The listing builds one solid part. Answer for the finished solid, in the listing's coordinates (mm). A direction names the side the tool comes from. Coordinates: 2 decimals unless noted, no trailing zeros. Write each loop counter-clockwise with the first axis right and the second up, starting at its lowest first coordinate (ties: lowest second). Pieces come first, ordered by that corner, then holes. Notation, with made-up numbers: M 54,22 L 95,22 A12 cw 95,45 Z; hole C 79,37.5 d11. An arc over 180 degrees is marked long. Write item = value, one per line. Start each with the question number.
```python
from build123d import *

# Parameters (mm, degrees)
SKETCH1_W                      = 65
SKETCH1_H                      = 32
EXTRUDE1_DEPTH                 = 6.35
CBORE_FOR_M4_SHCS1_D           = 4.5
CBORE_FOR_M4_SHCS1_CBORE_D     = 8
CBORE_FOR_M4_SHCS1_CBORE_DEPTH = 4
LPATTERN2_COUNT                = 2
LPATTERN2_PITCH                = 58
LPATTERN2_COUNT_DIR2           = 2
LPATTERN2_PITCH_DIR2           = 25
CBORE_FOR_M3_SHCS1_D           = 3.4
CBORE_FOR_M3_SHCS1_CBORE_D     = 6.5
CBORE_FOR_M3_SHCS1_CBORE_DEPTH = 4
LPATTERN3_COUNT                = 2
LPATTERN3_PITCH                = 16.2
LPATTERN3_COUNT_DIR2           = 2
LPATTERN3_PITCH_DIR2           = 25.4
LPATTERN4_COUNT                = 2
LPATTERN4_PITCH                = 25


with BuildPart() as part:
    # Sketch1 → Extrude1 (new body)
    with BuildSketch(Plane(origin=(0, 0, 0), x_dir=(1, 0, 0), z_dir=(0, 1, 0))):
        Rectangle(SKETCH1_W, SKETCH1_H)
    extrude(amount=EXTRUDE1_DEPTH)

    # CBORE for M4 SHCS1 (through all)
    with Locations(Plane(origin=(-29, 6.35, -12.5), x_dir=(0, 0, 1), z_dir=(0, 1, 0))):
        with Locations((0, 0)):
            cbore_for_m4_shcs1 = CounterBoreHole(CBORE_FOR_M4_SHCS1_D / 2, CBORE_FOR_M4_SHCS1_CBORE_D / 2, CBORE_FOR_M4_SHCS1_CBORE_DEPTH)

    # LPattern2: CBORE for M4 SHCS1 2 × 2
    with Locations(*[(i * LPATTERN2_PITCH, 0, j * LPATTERN2_PITCH_DIR2) for i in range(LPATTERN2_COUNT) for j in range(LPATTERN2_COUNT_DIR2) if (i, j) != (0, 0)]):
        add(cbore_for_m4_shcs1, mode=Mode.SUBTRACT)

    # CBORE for M3 SHCS1 (through all)
    with Locations(Plane(origin=(-8.1, 0, 12.7), x_dir=(0, 0, -1), z_dir=(0, -1, 0))):
        with Locations((0, 0)):
            cbore_for_m3_shcs1 = CounterBoreHole(CBORE_FOR_M3_SHCS1_D / 2, CBORE_FOR_M3_SHCS1_CBORE_D / 2, CBORE_FOR_M3_SHCS1_CBORE_DEPTH)

    # LPattern3: CBORE for M3 SHCS1 2 × 2
    with Locations(*[(i * LPATTERN3_PITCH, 0, -j * LPATTERN3_PITCH_DIR2) for i in range(LPATTERN3_COUNT) for j in range(LPATTERN3_COUNT_DIR2) if (i, j) != (0, 0)]):
        add(cbore_for_m3_shcs1, mode=Mode.SUBTRACT)

    # Sketch8 → Ø3.1 (3.1) Diameter Hole1 (revolve, cut)
    with BuildSketch(Plane(origin=(-12.5, 6.35, 0), x_dir=(0, 0, 1), z_dir=(1, 0, 0))):
        Polygon((0, 0), (0, 5.931333959), (1.55, 5), (1.55, 0), align=None)
    f_3_1_3_1_diameter_hole1 = revolve(axis=Axis((-12.5, 12.7, 0), (0, -1, 0)), mode=Mode.SUBTRACT)

    # LPattern4: Ø3.1 (3.1) Diameter Hole1 ×2
    with Locations(*[(i * LPATTERN4_PITCH, 0, 0) for i in range(1, LPATTERN4_COUNT)]):
        add(f_3_1_3_1_diameter_hole1, mode=Mode.SUBTRACT)


solid = part.part
```
1. Each of these flat-tipped pins is pushed along its axis until it touches: pin 1 (6 mm diameter, centred on x = -25, z = -3, fed in from -Y); pin 2 (2 mm diameter, centred on x = 27.5, z = 11, fed in from +Y); pin 3 (6 mm diameter, centred on x = -8.1, z = -12.7, fed in from -Y). Where does it stop, or does it pass through?
2. For faces 4 (the face through (32.1, 6.35, -15.6)), 5 (the face through (-7.12, 1.97, -15.8)), 6 (the face through (26.099, 4.378, -9.746)), determine the directions among +Z, -Z, +X, -X, +Y, -Y from which every point of the face is accessible in a straight line to the end or side of a thin tool.
3. Straight lines are drawn through the part: L1, parallel to X at y = 2, z = -12.7; L2, parallel to X at y = 3, z = -12.5; L3, parallel to X at y = 3, z = -0.5. For each, find the intervals that lie inside material, in ascending order. Write a range as [from, to].
4. For a pull along Z with two mould halves and no side action, classify faces 1 (the face through (0, 0, 0)), 2 (the face through (0, 3, -16)), 3 (the face through (7, 4, 11)) as pulls with the +Z half, pulls with the -Z half, needs draft (parallel to the pull), parting line crosses it, or undercut.
5. The part is cut by section A-A, the plane x = 29. Write down the section's boundary in (y, z), and give its area (3 significant figures).
6. The part is cut by section B-B, the plane z = -12.7. Count the separate pieces of the cut face and the enclosed holes in it, and give its area (3 significant figures).
Solution:
q1.pin_1 = 0
q1.pin_2 = 2.35
q1.pin_3 = 4
q2.face_4 = +Z, -Z, +X, -X, +Y
q2.face_5 = -Y
q2.face_6 = +Y
q3.L1 = [-32.5, -31.24], [-26.76, -11.35], [-4.85, 4.85], [11.35, 26.76], [31.24, 32.5]
q3.L2 = [-25, -11.34], [-4.86, 4.86], [11.34, 25]
q3.L3 = [-32.5, -13.97], [-11.03, 11.03], [13.97, 32.5]
q4.face_1 = needs draft
q4.face_2 = pulls with the -Z half
q4.face_3 = undercut
q5.outline = M 0,-16 L 2.35,-16 L 2.35,-14.75 L 0,-14.75 Z; M 0,-10.25 L 2.35,-10.25 L 2.35,-8.5 L 6.35,-8.5 L 6.35,8.5 L 2.35,8.5 L 2.35,10.25 L 0,10.25 Z; M 0,14.75 L 2.35,14.75 L 2.35,16 L 0,16 Z
q5.area = 122 mm^2
q6.separate_pieces = 5
q6.enclosed_holes = 0
q6.area = 264 mm^2
